Design review of the part shown in the three views and the two pictorial views. Dimensions are in mm from the part's minimum x, y and z. A direction names the side the tool comes from. Give positions to 0.01 mm unless a question says otherwise; leave off trailing zeros. Write each loop counter-clockwise with the first axis right and the second up, starting at its lowest first coordinate (ties: lowest second). Pieces come first, ordered by that corner, then holes. Notation, with made-up numbers: M -12,57 L 18,57 A14 ccw 18,61 Z; hole C 36.5,89.25 d6. An arc over 180 degrees is marked long. Write item = value, one per line.
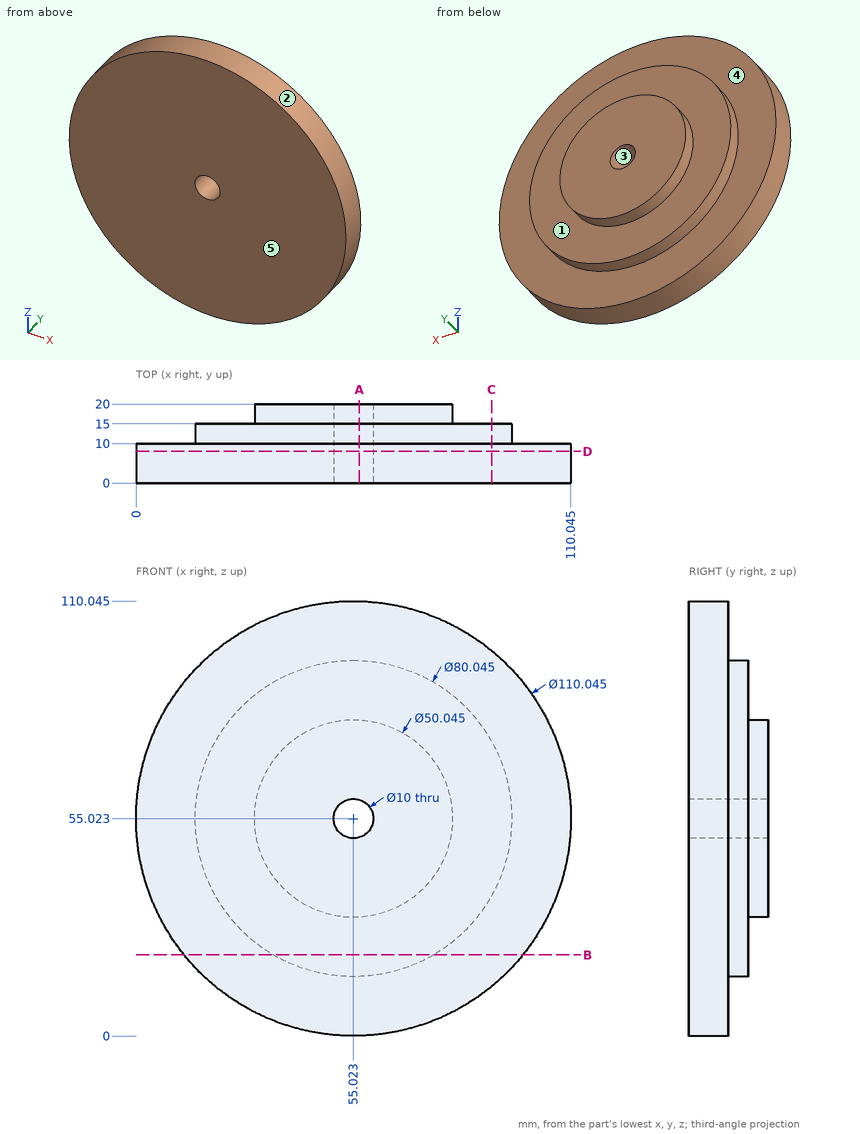
1. For line 1 along Y through (x, z) = (73, 33.5); line 2 along Z through (x, y) = (56.5, 8.5) (1 decimal); line 3 along Y through (x, z) = (98.5, 26.5), list the stretches that pass through material, from the lowest coordinate up. Write a range as from..to.
Responses:
line_1 = 0..15
line_2 = 0..50.2, 59.8..110
line_3 = 0..10
2. Machinability: for the marked faces 4 and 5, which of the approach directions +Z, -Z, +X, -X, +Y, -Y give a long, thin tool a straight path to every point of the face, cutting with its end or side? Answer none if there is none.
Responses:
face_4 = +Y
face_5 = +Z, -Z, +X, -X, -Y
3. We need section A-A, the plane x = 56.5. Write out the cut boundary in (y, z) (1 decimal).
Responses:
outline = M 0,0 L 10,0 L 10,15 L 15,15 L 15,30 L 20,30 L 20,50.2 L 0,50.2 Z; M 0,59.8 L 20,59.8 L 20,80 L 15,80 L 15,95 L 10,95 L 10,110 L 0,110 Z
4. The part is to be moulded in two halves that separate along Z. For the marked faces 1, 2 and 3, say which applies: +Z half, -Z half, draft (parallel to the pull), parting line (faces both ways), or undercut.
Responses:
face_1 = draft
face_2 = parting line
face_3 = undercut
5. We need section B-B, the plane z = 20.5. Write out the cut boundary in (x, y) (1 decimal).
Responses:
outline = M 12.2,0 L 97.9,0 L 97.9,10 L 75.3,10 L 75.3,15 L 34.8,15 L 34.8,10 L 12.2,10 Z
6. Insertion check: P1, Ø10, axis at y = 8.5, z = 77, coming from the -X side (1 decimal); P2, Ø1, axis at x = 89, y = 11, coming from the -Z side; P3, Ø5, axis at x = 14, y = 6.5, coming from the +Z side; P4, Ø13, axis at x = 55.02, z = 55.02, coming from the -Y side. Each pin has a flat end and moves straight along its axis. Give the tip position at first contact, or say it passes through.
Responses:
P1 = 2.7
P2 = 33.09
P3 = 94.31
P4 = 0
7. We need section D-D, the plane y = 8. Write out the cut boundary in (x, z) (1 decimal).
Responses:
outline = C 55,55 d110; hole C 55,55 d10
8. We need section C-C, the plane x = 90. Write out the cut boundary in (y, z) (1 decimal), then the cut area to 3 significant figures.
Responses:
outline = M 0,12.5 L 10,12.5 L 10,35.6 L 15,35.6 L 15,74.5 L 10,74.5 L 10,97.5 L 0,97.5 Z
area = 1,040 mm2
